Model file for the job. Use its own axes, mm. Coordinates: 2 decimals unless noted, no trailing zeros. Write each loop counter-clockwise with the first axis right and the second up, starting at its lowest first coordinate (ties: lowest second). Pieces come first, ordered by that corner, then holes. Notation, with made-up numbers: M 24,44 L 45,44 A27 ccw 45,79 Z; hole C -20.75,4 d2. An arc over 180 degrees is marked long. Put each result on its own line as item: value. Start each with the question number.
Q1. Drill centre lines: line 1 along Y through (x, z) = (33, 1.7); line 2 along Y through (x, z) = (55, 2.5); line 3 along X through (y, z) = (45.75, 3). Where is each one in solid material? Low to high.
Q2. Cut at C-C (x = -101.41). Write the cut outline in (y, z), then the cut area to 3 significant figures.
Q3. Cut at A-A (x = 33). Write the cut outline in (y, z), then the cut area to 3 significant figures.
Q4. Drop flat-ended pins along their axis: pin 1 (3 mm diameter, centred on x = 40.5, y = -33, fed in from -Z); pin 2 (1 mm diameter, centred on y = 25, z = 0.5, fed in from -X); pin 3 (3 mm diameter, centred on x = 0, y = -42.76, fed in from +Z); pin 4 (1.5 mm diameter, centred on x = -138, z = 5, fed in from -Y). Give the stop position or say it passes through.
Q5. Cut at B-B (x = -57). Write the cut outline in (y, z), then the cut area to 3 significant figures.
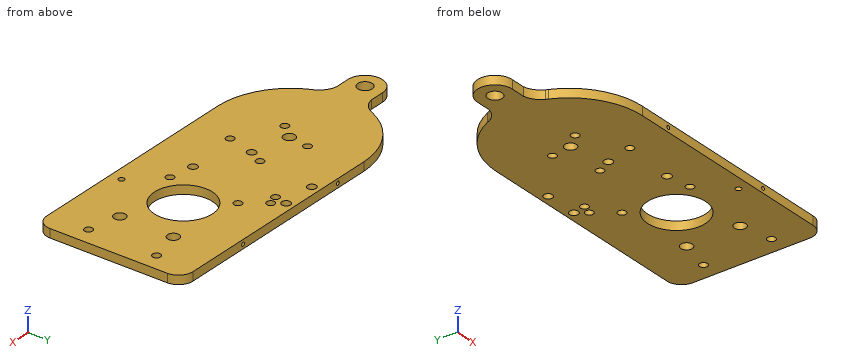
```python
from build123d import *

# Parameters (mm, degrees)
F0_R     = 5
F0_R_2   = 2.75
F0_R_3   = 3
F0_R_4   = 2
F0_R_5   = 20
F0_R_6   = 4
F1_DEPTH = 6
F4_D     = 2.5
F4_DEPTH = 7.6
F4_TIP   = 0.7510757738
F7_D     = 2.5
F7_DEPTH = 7.6
F7_TIP   = 0.7510757738


with BuildPart() as f1:
    # F0 (on Top) → F1 (new body)
    with BuildSketch(Plane.XY):
        with BuildLine():
            Line((57, 50.5), (-96.28, 50.5))
            ThreePointArc((-96.28, 50.5), (-123.5701507697, 42.4911481484), (-142.2043500731, 21.0048582562))
            ThreePointArc((-142.2043500731, 21.0048582562), (-142.5276249328, 20.1970602892), (-142.900454883, 19.4109038043))
            ThreePointArc((-142.900454883, 19.4109038043), (-147.0751075285, 14.512842569), (-153, 12))
            Line((-153, 12), (-163, 12))
            ThreePointArc((-163, 12), (-175, 0), (-163, -12))
            Line((-163, -12), (-153, -12))
            ThreePointArc((-153, -12), (-147.0751075285, -14.512842569), (-142.900454883, -19.4109038043))
            ThreePointArc((-142.900454883, -19.4109038043), (-142.5276249328, -20.1970602892), (-142.2043500731, -21.0048582562))
            ThreePointArc((-142.2043500731, -21.0048582562), (-123.5701507697, -42.4911481484), (-96.28, -50.5))
            Line((-96.28, -50.5), (57, -50.5))
            ThreePointArc((57, -50.5), (64.0710678119, -47.5710678119), (67, -40.5))
            Line((67, -40.5), (67, 40.5))
            ThreePointArc((67, 40.5), (64.0710678119, 47.5710678119), (57, 50.5))
        make_face()
        with Locations((-163, 0)):
            Circle(F0_R, mode=Mode.SUBTRACT)
        with Locations((-72, -23.2)):
            Circle(F0_R_2, mode=Mode.SUBTRACT)
        with Locations((-101.41, -8)):
            Circle(F0_R_2, mode=Mode.SUBTRACT)
        with Locations((-67.15, -4.55)):
            Circle(F0_R_3, mode=Mode.SUBTRACT)
        with Locations((0, -42.7629426122)):
            Circle(F0_R_4, mode=Mode.SUBTRACT)
        with Locations((-35, -20.3005317599)):
            Circle(F0_R_3, mode=Mode.SUBTRACT)
        with Locations((-18, -23.2)):
            Circle(F0_R_2, mode=Mode.SUBTRACT)
        Circle(F0_R_5, mode=Mode.SUBTRACT)
        with Locations((33, -18.5)):
            Circle(F0_R_6, mode=Mode.SUBTRACT)
        with Locations((55, -23.2)):
            Circle(F0_R_2, mode=Mode.SUBTRACT)
        with Locations((-93.1177586317, 1.52)):
            Circle(F0_R_6, mode=Mode.SUBTRACT)
        with Locations((-62.2, 5)):
            Circle(F0_R_2, mode=Mode.SUBTRACT)
        with Locations((-91.15, 15.6)):
            Circle(F0_R_2, mode=Mode.SUBTRACT)
        with Locations((-57, 44.8)):
            Circle(F0_R_3, mode=Mode.SUBTRACT)
        with Locations((-18, 23.8)):
            Circle(F0_R_2, mode=Mode.SUBTRACT)
        with Locations((33, 18.5)):
            Circle(F0_R_6, mode=Mode.SUBTRACT)
        with Locations((55, 23.8)):
            Circle(F0_R_2, mode=Mode.SUBTRACT)
        with Locations((-35.9, 36)):
            Circle(F0_R_2, mode=Mode.SUBTRACT)
        with Locations((-29, 38)):
            Circle(F0_R_2, mode=Mode.SUBTRACT)
        with Locations((-34, 44.8)):
            Circle(F0_R_3, mode=Mode.SUBTRACT)
    extrude(amount=F1_DEPTH)

    # F4
    with Locations(Plane.XZ.offset(50.5)):
        with Locations((-73, 3), (12, 3)):
            Hole(F4_D / 2, depth=F4_DEPTH)
            with Locations((0, 0, -(F4_DEPTH + F4_TIP / 2))):  # 118° drill point
                Cone(0, F4_D / 2, F4_TIP, mode=Mode.SUBTRACT)

    # F7
    with Locations(Plane(origin=(0, 50.5, 0), x_dir=(-1, 0, 0), z_dir=(0, 1, 0))):
        with Locations((-12, 3), (73, 3)):
            Hole(F7_D / 2, depth=F7_DEPTH)
            with Locations((0, 0, -(F7_DEPTH + F7_TIP / 2))):  # 118° drill point
                Cone(0, F7_D / 2, F7_TIP, mode=Mode.SUBTRACT)


solid = f1.part
```
Computed values:
1. line 1: -50.5 to -22.5, -14.5 to 14.5, 22.5 to 50.5
1. line 2: -50.5 to -25.95, -20.45 to 21.05, 26.55 to 50.5
1. line 3: -117.66 to -74.25, -71.75 to -59.85, -54.15 to -36.85, -31.15 to 10.75, 13.25 to 65.51
2. outline: M -50.24,0 L -10.75,0 L -10.75,6 L -50.24,6 Z; M -5.25,0 L 50.24,0 L 50.24,6 L -5.25,6 Z
2. area: 570 mm2
3. outline: M -50.5,0 L -22.5,0 L -22.5,6 L -50.5,6 Z; M -14.5,0 L 14.5,0 L 14.5,6 L -14.5,6 Z; M 22.5,0 L 50.5,0 L 50.5,6 L 22.5,6 Z
3. area: 510 mm2
4. pin 1: z = 0
4. pin 2: x = -140.44
4. pin 3: through
4. pin 4: y = -29.52
5. outline: M -50.5,0 L 41.8,0 L 41.8,6 L -50.5,6 Z; M 47.8,0 L 50.5,0 L 50.5,6 L 47.8,6 Z
5. area: 570 mm2
